Read the model definition and answer for the solid it produces. Units are mm, in the model's axes. Face numbers are marked on the shaded views. A direction names the side the tool comes from. Give positions to 0.01 mm unless a question says otherwise; leave off trailing zeros. Loops run counter-clockwise (first coordinate to the right, second up) from the corner with the lowest first, then second, coordinate; pieces in that order, holes last. Notation, with made-up numbers: M 49.5,-18.5 L 58.5,-18.5 A16 cw 58.5,0.5 Z; hole C -39.5,38.5 d7. An arc over 180 degrees is marked long. Return JSON: item names as keys, results as strings. Group by question number.
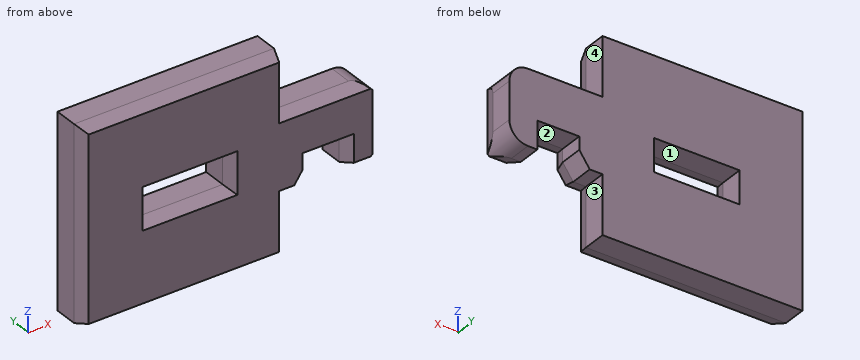
```python
from build123d import *
from OCP.BRepFilletAPI import BRepFilletAPI_MakeChamfer

# Parameters (mm, degrees)
SKETCH1_W           = 21.447515714
SKETCH1_H           = 20.590988136
SKETCH1_W_2         = 9.2
SKETCH1_H_2         = 3.53
BOSS_EXTRUDE1_DEPTH = 4
SKETCH2_W           = 10
SKETCH2_H           = 8
BOSS_EXTRUDE3_DEPTH = 4
CUT_EXTRUDE1_DEPTH  = 24.022536743
CHAMFER1_SIZE       = 1.5
CHAMFER1_SIZE2      = 0.5
FILLET1_R           = 2


with BuildPart() as part:
    # Sketch1 → Boss-Extrude1 (new body)
    with BuildSketch(Plane(origin=(0, 0, 0), x_dir=(1, 0, 0), z_dir=(0, 1, 0))):
        with Locations((-0.523757857, 0)):
            Rectangle(SKETCH1_W, SKETCH1_H)
        with Locations((0.1, 0)):
            Rectangle(SKETCH1_W_2, SKETCH1_H_2, mode=Mode.SUBTRACT)
    extrude(amount=BOSS_EXTRUDE1_DEPTH)

    # Sketch2 → Boss-Extrude3 (add)
    with BuildSketch(Plane(origin=(0, 0, 0), x_dir=(1, 0, 0), z_dir=(0, 1, 0))):
        with Locations((15.2, 0)):
            Rectangle(SKETCH2_W, SKETCH2_H)
    extrude(amount=BOSS_EXTRUDE3_DEPTH)

    # Sketch3 → Cut-Extrude1 (cut, through all)
    with BuildSketch(Plane(origin=(0, 0, 0), x_dir=(1, 0, 0), z_dir=(0, 1, 0))):
        Polygon((12.7, 1), (12.7, 2.38454447), (11.576199706, 4), (12.7, 4), (17.2, 4), (17.2, 1), align=None)
    extrude(amount=CUT_EXTRUDE1_DEPTH, mode=Mode.SUBTRACT)

    # Chamfer1: one chamfer whose edges measure the first distance from different faces: ONE call of the kernel's chamfer builder (chamfer() names one face for all edges)
    chamfer1_edges_1 = [part.edges().sort_by_distance(p)[0] for p in [
        (4.7, 0, 0),
    ]]
    chamfer1_side_1 = [part.faces().sort_by_distance(p)[0] for p in [
        (4.7, 2, 0),
    ]]
    chamfer1_edges_2 = [part.edges().sort_by_distance(p)[0] for p in [
        (0.1, 0, -1.765),
    ]]
    chamfer1_side_2 = [part.faces().sort_by_distance(p)[0] for p in [
        (0.1, 2, -1.765),
    ]]
    chamfer1_edges_3 = [part.edges().sort_by_distance(p)[0] for p in [
        (-4.5, 0, 0),
    ]]
    chamfer1_side_3 = [part.faces().sort_by_distance(p)[0] for p in [
        (-4.5, 2, 0),
    ]]
    chamfer1_edges_4 = [part.edges().sort_by_distance(p)[0] for p in [
        (0.1, 0, 1.765),
    ]]
    chamfer1_side_4 = [part.faces().sort_by_distance(p)[0] for p in [
        (0.1, 2, 1.765),
    ]]
    chamfer1_edges_5 = [part.edges().sort_by_distance(p)[0] for p in [
        (10.2, 0, -7.147747034),
    ]]
    chamfer1_side_5 = [part.faces().sort_by_distance(p)[0] for p in [
        (10.2, 2, -7.147747034),
    ]]
    chamfer1_edges_6 = [part.edges().sort_by_distance(p)[0] for p in [
        (15.2, 0, 4),
    ]]
    chamfer1_side_6 = [part.faces().sort_by_distance(p)[0] for p in [
        (15.2, 2, 4),
    ]]
    chamfer1_edges_7 = [part.edges().sort_by_distance(p)[0] for p in [
        (20.2, 0, 0),
    ]]
    chamfer1_side_7 = [part.faces().sort_by_distance(p)[0] for p in [
        (20.2, 2, 0),
    ]]
    chamfer1_edges_8 = [part.edges().sort_by_distance(p)[0] for p in [
        (18.7, 0, -4),
    ]]
    chamfer1_side_8 = [part.faces().sort_by_distance(p)[0] for p in [
        (18.7, 2, -4),
    ]]
    chamfer1_edges_9 = [part.edges().sort_by_distance(p)[0] for p in [
        (10.888099853, 0, -4),
    ]]
    chamfer1_side_9 = [part.faces().sort_by_distance(p)[0] for p in [
        (10.888099853, 2, -4),
    ]]
    chamfer1_edges_10 = [part.edges().sort_by_distance(p)[0] for p in [
        (12.138099853, 0, -3.192272235),
    ]]
    chamfer1_side_10 = [part.faces().sort_by_distance(p)[0] for p in [
        (12.138099853, 2, -3.192272235),
    ]]
    chamfer1_edges_11 = [part.edges().sort_by_distance(p)[0] for p in [
        (12.7, 0, -1.692272235),
    ]]
    chamfer1_side_11 = [part.faces().sort_by_distance(p)[0] for p in [
        (12.7, 2, -1.692272235),
    ]]
    chamfer1_edges_12 = [part.edges().sort_by_distance(p)[0] for p in [
        (14.95, 0, -1),
    ]]
    chamfer1_side_12 = [part.faces().sort_by_distance(p)[0] for p in [
        (14.95, 2, -1),
    ]]
    chamfer1_edges_13 = [part.edges().sort_by_distance(p)[0] for p in [
        (17.2, 0, -2.5),
    ]]
    chamfer1_side_13 = [part.faces().sort_by_distance(p)[0] for p in [
        (17.2, 2, -2.5),
    ]]
    chamfer1_edges_14 = [part.edges().sort_by_distance(p)[0] for p in [
        (-0.523757857, 0, -10.295494068),
    ]]
    chamfer1_side_14 = [part.faces().sort_by_distance(p)[0] for p in [
        (-0.523757857, 2, -10.295494068),
    ]]
    chamfer1_edges_15 = [part.edges().sort_by_distance(p)[0] for p in [
        (10.2, 0, 7.147747034),
    ]]
    chamfer1_side_15 = [part.faces().sort_by_distance(p)[0] for p in [
        (10.2, 2, 7.147747034),
    ]]
    chamfer1_edges_16 = [part.edges().sort_by_distance(p)[0] for p in [
        (-0.523757857, 0, 10.295494068),
    ]]
    chamfer1_side_16 = [part.faces().sort_by_distance(p)[0] for p in [
        (-0.523757857, 2, 10.295494068),
    ]]
    chamfer1_edges_17 = [part.edges().sort_by_distance(p)[0] for p in [
        (-11.247515714, 0, 0),
    ]]
    chamfer1_side_17 = [part.faces().sort_by_distance(p)[0] for p in [
        (-11.247515714, 2, 0),
    ]]
    chamfer1 = BRepFilletAPI_MakeChamfer(part.part.solid().wrapped)
    for e in chamfer1_edges_1:
        chamfer1.Add(CHAMFER1_SIZE, CHAMFER1_SIZE2, e.wrapped, chamfer1_side_1[0].wrapped)  # the first distance lies on this face
    for e in chamfer1_edges_2:
        chamfer1.Add(CHAMFER1_SIZE, CHAMFER1_SIZE2, e.wrapped, chamfer1_side_2[0].wrapped)  # the first distance lies on this face
    for e in chamfer1_edges_3:
        chamfer1.Add(CHAMFER1_SIZE, CHAMFER1_SIZE2, e.wrapped, chamfer1_side_3[0].wrapped)  # the first distance lies on this face
    for e in chamfer1_edges_4:
        chamfer1.Add(CHAMFER1_SIZE, CHAMFER1_SIZE2, e.wrapped, chamfer1_side_4[0].wrapped)  # the first distance lies on this face
    for e in chamfer1_edges_5:
        chamfer1.Add(CHAMFER1_SIZE, CHAMFER1_SIZE2, e.wrapped, chamfer1_side_5[0].wrapped)  # the first distance lies on this face
    for e in chamfer1_edges_6:
        chamfer1.Add(CHAMFER1_SIZE, CHAMFER1_SIZE2, e.wrapped, chamfer1_side_6[0].wrapped)  # the first distance lies on this face
    for e in chamfer1_edges_7:
        chamfer1.Add(CHAMFER1_SIZE, CHAMFER1_SIZE2, e.wrapped, chamfer1_side_7[0].wrapped)  # the first distance lies on this face
    for e in chamfer1_edges_8:
        chamfer1.Add(CHAMFER1_SIZE, CHAMFER1_SIZE2, e.wrapped, chamfer1_side_8[0].wrapped)  # the first distance lies on this face
    for e in chamfer1_edges_9:
        chamfer1.Add(CHAMFER1_SIZE, CHAMFER1_SIZE2, e.wrapped, chamfer1_side_9[0].wrapped)  # the first distance lies on this face
    for e in chamfer1_edges_10:
        chamfer1.Add(CHAMFER1_SIZE, CHAMFER1_SIZE2, e.wrapped, chamfer1_side_10[0].wrapped)  # the first distance lies on this face
    for e in chamfer1_edges_11:
        chamfer1.Add(CHAMFER1_SIZE, CHAMFER1_SIZE2, e.wrapped, chamfer1_side_11[0].wrapped)  # the first distance lies on this face
    for e in chamfer1_edges_12:
        chamfer1.Add(CHAMFER1_SIZE, CHAMFER1_SIZE2, e.wrapped, chamfer1_side_12[0].wrapped)  # the first distance lies on this face
    for e in chamfer1_edges_13:
        chamfer1.Add(CHAMFER1_SIZE, CHAMFER1_SIZE2, e.wrapped, chamfer1_side_13[0].wrapped)  # the first distance lies on this face
    for e in chamfer1_edges_14:
        chamfer1.Add(CHAMFER1_SIZE, CHAMFER1_SIZE2, e.wrapped, chamfer1_side_14[0].wrapped)  # the first distance lies on this face
    for e in chamfer1_edges_15:
        chamfer1.Add(CHAMFER1_SIZE, CHAMFER1_SIZE2, e.wrapped, chamfer1_side_15[0].wrapped)  # the first distance lies on this face
    for e in chamfer1_edges_16:
        chamfer1.Add(CHAMFER1_SIZE, CHAMFER1_SIZE2, e.wrapped, chamfer1_side_16[0].wrapped)  # the first distance lies on this face
    for e in chamfer1_edges_17:
        chamfer1.Add(CHAMFER1_SIZE, CHAMFER1_SIZE2, e.wrapped, chamfer1_side_17[0].wrapped)  # the first distance lies on this face
    add(Compound.cast(chamfer1.Shape()), mode=Mode.REPLACE)

    # Fillet1
    # the kernel refuses this fillet: 2 mm, written as the material it takes off along each edge
    with BuildSketch(Plane(origin=(20.2, -3.5, 4), x_dir=(-1, 0, 0), z_dir=(0, 1, 0)), Plane(origin=(20.2, -3.5, -4), x_dir=(0, 0, 1), z_dir=(0, 1, 0))) as fillet1_piece_1:
        with BuildLine():
            CenterArc((FILLET1_R, -FILLET1_R), FILLET1_R, 90, 90)
            Line((0, -FILLET1_R), (0, 0))
            Line((0, 0), (FILLET1_R, 0))
        make_face()
    extrude(amount=12.5, mode=Mode.SUBTRACT)


solid = part.part
```
1. For the marked faces 1, 2, 3 and 4, determine the directions among +Z, -Z, +X, -X, +Y, -Y from which every point of the face is accessible in a straight line to the end or side of a thin tool.
2. Find section A-A (z = 0). Write down the section's boundary in (x, y), and give its area (3 significant figures).
3. Straight lines are drawn through the part: line 1 along X through (y, z) = (2.15, -1.25); line 2 along X through (y, z) = (1.8, 0); line 3 along Z through (x, y) = (-2, 3.65) (1 decimal). For each, find the intervals that lie inside material, in ascending order.
4. Find section C-C (y = 2.45). Write down the section's boundary in (x, z) (1 decimal), and give its area (3 significant figures).
5. Flat-ended cylindrical pins translate along their axes: P1, Ø1.5, axis at x = 11, y = 2.5, coming from the -Z side; P2, Ø1, axis at x = 16.5, y = 1.5, coming from the -Z side; P3, Ø5, axis at x = 4, z = 0, coming from the +Y side; P4, Ø0.8, axis at y = 3, z = 7.5, coming from the +X side. Find the tip coordinate at first contact, or state that the pin passes through.
6. Find section D-D (z = 5). Write down the section's boundary in (x, y), and give its area (3 significant figures).
7. Find section B-B (x = -4). Write down the section's boundary in (y, z) (1 decimal).
Result:
{
 "1": {"face 1": "+Y, -Y", "face 2": "-Z, +Y, -Y", "face 3": "-Z, +X, +Y, -Y", "face 4": "+Z, +X, +Y, -Y"},
 "2": {"outline": "M -11.25,1.5 L -10.75,0 L -5,0 L -4.5,1.5 L -4.5,4 L -11.25,4 Z; M 4.7,1.5 L 5.2,0 L 19.7,0 L 20.2,1.5 L 20.2,4 L 4.7,4 Z", "area": "87.5 mm2"},
 "3": {"line 1": "x = -11.25 to -4.5, 4.7 to 12.7, 17.2 to 20.2", "line 2": "x = -11.25 to -4.5, 4.7 to 20.2", "line 3": "z = -10.3 to -1.8, 1.8 to 10.3"},
 "4": {"outline": "M -11.2,-10.3 L 10.2,-10.3 L 10.2,-4 L 11.6,-4 L 12.7,-2.4 L 12.7,-1 L 17.2,-1 L 17.2,-4 L 18.2,-4 A2 ccw 20.2,-2 L 20.2,2 A2 ccw 18.2,4 L 10.2,4 L 10.2,10.3 L -11.2,10.3 Z; hole M -4.5,-1.8 L 4.7,-1.8 L 4.7,1.8 L -4.5,1.8 Z", "area": "473 mm2"},
 "5": {"P1": "stops at z = -4", "P2": "stops at z = -1", "P3": "stops at y = 4", "P4": "stops at x = 10.2"},
 "6": {"outline": "M -11.25,1.5 L -10.75,0 L 9.7,0 L 10.2,1.5 L 10.2,4 L -11.25,4 Z", "area": "85.0 mm2"},
 "7": {"outline": "M 0,-9.8 L 1.5,-10.3 L 4,-10.3 L 4,-1.8 L 1.5,-1.8 L 0,-2.3 Z; M 0,2.3 L 1.5,1.8 L 4,1.8 L 4,10.3 L 1.5,10.3 L 0,9.8 Z"}
}
